from build123d import *

# Parameters (mm, degrees)
F0_W     = 88
F0_H     = 88
F1_DEPTH = 50
F2_W     = 22.5
F2_H     = 4
F2_W_2   = 12
F2_H_2   = 2
F3_DEPTH = 17.5


with BuildPart() as f1:
    # F0 (on Top) → F1 (new body)
    with BuildSketch(Plane.XY):
        with Locations((4.011764, -4.715418)):
            Rectangle(F0_W, F0_H)
    extrude(amount=F1_DEPTH)

    # F2 (on face) → F3 (cut)
    with BuildSketch(Plane.XY.offset(50)):
        with Locations((-23.445669, 29.813612)):
            Rectangle(F2_W, F2_H)
        with Locations((-23.445669, 17.113612)):
            Rectangle(F2_W, F2_H)
        with Locations((-23.445669, 4.413612)):
            Rectangle(F2_W, F2_H)
        with Locations((-23.445669, -8.286388)):
            Rectangle(F2_W, F2_H)
        with Locations((-23.445669, -20.986388)):
            Rectangle(F2_W, F2_H)
        with Locations((-23.445669, -33.686388)):
            Rectangle(F2_W, F2_H)
        with Locations((-23.445669, -46.386388)):
            Rectangle(F2_W, F2_H)
        with Locations((17.377627, 28.813612)):
            Rectangle(F2_W_2, F2_H_2)
        with Locations((17.377627, 16.113612)):
            Rectangle(F2_W_2, F2_H_2)
        with Locations((17.377627, 3.413612)):
            Rectangle(F2_W_2, F2_H_2)
        with Locations((17.377627, -9.286388)):
            Rectangle(F2_W_2, F2_H_2)
        with Locations((17.377627, -21.986388)):
            Rectangle(F2_W_2, F2_H_2)
        with Locations((17.377627, -34.686388)):
            Rectangle(F2_W_2, F2_H_2)
        with Locations((17.377627, -47.386388)):
            Rectangle(F2_W_2, F2_H_2)
    extrude(amount=-F3_DEPTH, mode=Mode.SUBTRACT)


solid = f1.part
Design review of the part built by this model. Coordinates are the model's own, in mm. A direction names the side the tool comes from. Give positions to 0.01 mm unless a question says otherwise; leave off trailing zeros. Answer as a JSON object with one key per item and string values. Group by question number.
1) For line 1 along X through (y, z) = (-35, 37); line 2 along X through (y, z) = (-20.5, 44); line 3 along Z through (x, y) = (22.5, 28.5), list the stretches that pass through material, from the lowest coordinate up.
2) Tool access review of faces 1 (the face through (3, -4, 0)), 2 (the face through (-12.196, 17, 41)): name each direction out of +Z, -Z, +X, -X, +Y, -Y from which nothing blocks a thin tool from reaching the whole face with its end or side.
3) Clearance check with a flat-ended pin moving along its axis: pin 1 Ø0.6 at (x, y) = (20, -9.5) entering from +Z. State where the tip first meets the part, or that it passes through.
4) Mouldability with a two-part tool opening along Y and no side actions: class faces 3 (the face through (-24, -31.686, 41)), 4 (the face through (3, 39.285, 25)), 5 (the face through (-39.988, -5, 25)) as released by +Y, released by -Y, zero draft, split by the parting line, or undercut.
5) We need section A-A (z = 34). Count the separate pieces of the cut face and the enclosed holes in it, and give its area (3 significant figures).
Answer key:
{
 "1": {"line 1": "x = -39.99 to -34.7, -12.2 to 11.38, 23.38 to 48.01", "line 2": "x = -39.99 to -34.7, -12.2 to 48.01", "line 3": "z = 0 to 32.5"},
 "2": {"face 1": "-Z, +X, -X, +Y, -Y", "face 2": "+Z"},
 "3": {"pin 1": "stops at z = 32.5"},
 "4": {"face 3": "undercut", "face 4": "released by +Y", "face 5": "zero draft"},
 "5": {"separate pieces": "1", "enclosed holes": "14", "area": "6,950 mm²"}
}
